Design review of the part built by this model. Coordinates are the model's own, in mm. A direction names the side the tool comes from. Coordinates: 2 decimals unless noted, no trailing zeros. Order: outer loops, then holes, each group sorted by start corner. A loop starts at its lowest first (then second) coordinate and runs counter-clockwise, first axis right, second up. Notation, with made-up numbers: M 72,76 L 117,76 A24 ccw 117,109 Z; hole C -36,50 d1. An arc over 180 degrees is marked long. Answer in a Markdown table with one row per item.
from build123d import *

# Parameters (mm, degrees)
SKETCH1_R           = 1.6
BOSS_EXTRUDE1_DEPTH = 8.75
CHAMFER1_SIZE       = 0.4
CHAMFER1_SIZE2      = 0.571259203
SKETCH2_R           = 2.5
BOSS_EXTRUDE2_DEPTH = 2


with BuildPart() as part:
    # Sketch1 → Boss-Extrude1 (new, symmetric)
    with BuildSketch(Plane.XY):
        Circle(SKETCH1_R)
    extrude(amount=BOSS_EXTRUDE1_DEPTH, both=True)

    # Chamfer1
    chamfer1_edges = [part.edges().sort_by_distance(p)[0] for p in [
        (-1.6, 0, -8.75),
    ]]
    chamfer1_side = [part.faces().sort_by_distance(p)[0] for p in [
        (0, 0, -8.75),
    ]]
    chamfer(chamfer1_edges, length=CHAMFER1_SIZE, length2=CHAMFER1_SIZE2, reference=chamfer1_side[0])

    # Sketch2 → Boss-Extrude2 (add)
    with BuildSketch(Plane.XY.offset(8.75)):
        Circle(SKETCH2_R)
    extrude(amount=BOSS_EXTRUDE2_DEPTH)


solid = part.part
(1) For line 1 along Z through (x, y) = (1.1, -1.55); line 2 along Y through (x, z) = (0.25, 7); line 3 along X through (y, z) = (-1.05, -5), list the stretches that pass through material, from the lowest coordinate up. Write a range as from..to.
Return value:
| item | result |
|---|---|
| line 1 | z = 8.75..10.75 |
| line 2 | y = -1.58..1.58 |
| line 3 | x = -1.21..1.21 |
(2) Add section D-D, the plane z = 2.75. Give the boundary of the cut face in (x, y).
Return value:
| item | result |
|---|---|
| outline | C 0,0 d3.2 |
(3) Insertion check: pin 1 Ø3 at (x, z) = (0.5, 0.5) entering from -Y; pin 2 Ø3 at (x, z) = (-2, 4) entering from +Y. Each pin has a flat end and moves straight along its axis. Give the tip position at first contact, or say it passes through.
Return value:
| item | result |
|---|---|
| pin 1 | stops at y = -1.6 |
| pin 2 | stops at y = 1.52 |
(4) For faces 1 (the flat face through (0, -2, 8.75)), 2 (the flat face through (0, 0, 10.75)), list the 3-axis set-ups (+Z, -Z, +X, -X, +Y, -Y) from which the entire face can be reached by the end or side of a thin tool; tool diameter is ignored.
Return value:
| item | result |
|---|---|
| face 1 | -Z |
| face 2 | +Z, +X, -X, +Y, -Y |
(5) Add section C-C, the plane z = 9.5. Give the boundary of the cut face in (x, y).
Return value:
| item | result |
|---|---|
| outline | C 0,0 d5 |
(6) Add section A-A, the plane y = 0. Give the boundary of the cut face in (x, z), and give its area (3 significant figures).
Return value:
| item | result |
|---|---|
| outline | M -2.5,8.75 L -1.6,8.75 L -1.6,-8.18 L -1.2,-8.75 L 1.2,-8.75 L 1.6,-8.18 L 1.6,8.75 L 2.5,8.75 L 2.5,10.75 L -2.5,10.75 Z |
| area | 65.8 mm2 |
